Could you check a few things on this model? Use its own coordinates, in mm. A direction names the side the tool comes from. Coordinates: 2 decimals unless noted, no trailing zeros. Loops run counter-clockwise (first coordinate to the right, second up) from the corner with the lowest first, then second, coordinate; pieces in that order, holes last. Notation, with made-up numbers: M 2,51 L 17,51 A30 cw 17,75 Z; hole C 63,52 d2. An arc over 180 degrees is marked long. Use one line per item in the form item = value. Start each with the question number.
```python
from build123d import *

# Parameters (mm, degrees)
F1_DEPTH = 140
F2_T     = -2.5
F3_R     = 5


# Not quite as in the source:
# - a shell that OpenCascade refuses in one call is made with other operations: the cavity is built on its own and cut out


with BuildPart() as f1:
    # F0 (on Front) → F1 (new body)
    with BuildSketch(Plane.XZ):
        Polygon((-68.4042458236, 42.9600325577), (-68.4042458236, -74.0399674423), (61.5957541764, -74.0399674423), (61.5957541764, 42.9600325577), (38.1572941835, 42.9600325577), (38.1572941835, 15.1600325577), (-28.3427058165, 15.1600325577), (-28.3427058165, 42.9600325577), align=None)
    extrude(amount=F1_DEPTH)

    # F2: a shell. OpenCascade refuses it in one call, so the cavity is built on its own and cut out:
    # the body offset inwards by the wall thickness, plus a prism from it out through each open face.
    f2_core = offset(f1.part, amount=F2_T, kind=Kind.INTERSECTION, mode=Mode.PRIVATE)
    f2_exits = [f2_core.faces().sort_by_distance(p)[0] for p in [
        (4.907294, -70, 12.660033),
    ]]
    add(f2_core, mode=Mode.SUBTRACT)
    extrude(f2_exits, amount=-F2_T, mode=Mode.SUBTRACT)

    # F3
    f3_edges = [f1.edges().sort_by_distance(p)[0] for p in [
        (-68.404246, -70, 42.960033),
        (-68.404246, -70, -74.039967),
        (-68.404246, 0, -15.539967),
        (-68.404246, -140, -15.539967),
        (61.595754, -70, -74.039967),
        (61.595754, -70, 42.960033),
        (61.595754, 0, -15.539967),
        (61.595754, -140, -15.539967),
        (-3.404246, 0, -74.039967),
        (-3.404246, -140, -74.039967),
    ]]
    fillet(f3_edges, radius=F3_R)


solid = f1.part
```
Item 1: I want a section at D-D (y = -52). Write out the boundary of the cut face in (x, z), plus the area to 3 significant figures.
Item 2: I want a section at A-A (z = 34). Write out the boundary of the cut face in (x, y).
Item 3: I'm going to push flat-ended pins straight in: P1, Ø0.8, axis at x = 1.5, y = -1.5, coming from the +Z side; P2, Ø6, axis at x = -4.5, y = -99, coming from the +Z side. Where does each tip first touch, or does it pass through?
Item 4: Please list where these lines run through material, in increasing order: line 1 along X through (y, z) = (-25.5, 19); line 2 along Y through (x, z) = (55.5, -54); line 3 along Z through (x, y) = (-58, -131).
Item 5: Thinking about a two-plate mould opening in Z: for faces 1 (the flat face through (-4, -69, -71.54)), 2 (the flat face through (-28.343, -69, 29)), 3 (the flat face through (40.657, -69, 28)), 4 (the cylindrical face through (60.092, -70.91, -72.614)), which applies, pulls with the +Z half, pulls with the -Z half, needs draft (parallel to the pull), parting line crosses it, or undercut?
Item 6: For faces 5 (the flat face through (-46, -69, 42.96)), 6 (the flat face through (-65.904, -69, -15)), which set-ups out of +Z, -Z, +X, -X, +Y, -Y let a thin tool reach every point of the face, with its end or its side?
Item 7: I want a section at B-B (x = 51). Write out the boundary of the cut face in (y, z), plus the area to 3 significant figures.
Item 8: I want a section at C-C (x = -11.5). Write out the boundary of the cut face in (y, z), plus the area to 3 significant figures.
Worked answers:
q1.outline = M -68.4,-69.04 A5 ccw -63.4,-74.04 L 56.6,-74.04 A5 ccw 61.6,-69.04 L 61.6,37.96 A5 ccw 56.6,42.96 L 38.16,42.96 L 38.16,15.16 L 40.66,15.16 L 40.66,40.46 L 59.1,40.46 L 59.1,-71.54 L -65.9,-71.54 L -65.9,40.46 L -30.84,40.46 L -30.84,15.16 L -28.34,15.16 L -28.34,42.96 L -63.4,42.96 A5 ccw -68.4,37.96 Z
q1.area = 1,150 mm²
q2.outline = M -68.4,-135 A5 ccw -63.4,-140 L -28.34,-140 L -28.34,0 L -63.4,0 A5 ccw -68.4,-5 Z; M 38.16,-140 L 56.6,-140 A5 ccw 61.6,-135 L 61.6,-5 A5 ccw 56.6,0 L 38.16,0 Z; hole M -65.9,-137.5 L -30.84,-137.5 L -30.84,-2.5 L -65.9,-2.5 Z; hole M 40.66,-137.5 L 59.1,-137.5 L 59.1,-2.5 L 40.66,-2.5 Z
q3.P1 = 15.16
q3.P2 = -71.54
q4.line_1 = -68.4 to -65.9, -30.84 to -28.34, 38.16 to 40.66, 59.1 to 61.6
q4.line_2 = -140 to -137.5, -2.5 to 0
q4.line_3 = -74.04 to -71.54, 40.46 to 42.96
q5.face_1 = undercut
q5.face_2 = needs draft
q5.face_3 = undercut
q5.face_4 = pulls with the -Z half
q6.face_5 = +Z, +X, -X, +Y, -Y
q6.face_6 = none
q7.outline = M -140,-69.04 A5 ccw -135,-74.04 L -5,-74.04 A5 ccw 0,-69.04 L 0,42.96 L -140,42.96 Z; hole M -137.5,-71.54 L -2.5,-71.54 L -2.5,40.46 L -137.5,40.46 Z
q7.area = 1,250 mm²
q8.outline = M -140,-69.04 A5 ccw -135,-74.04 L -5,-74.04 A5 ccw 0,-69.04 L 0,15.16 L -2.5,15.16 L -2.5,-71.54 L -137.5,-71.54 L -137.5,15.16 L -140,15.16 Z
q8.area = 773 mm²
